from build123d import *
from build123d import SkipClean  # not in build123d's __all__

# Parameters (mm, degrees)
F0_W             = 44.45
F0_H             = 25.4
F1_DEPTH         = 44.45
F2_W             = 12.7
F2_H             = 44.45
F3_DEPTH         = 12.7
F4_W             = 44.45
F4_H             = 12.7
F5_DEPTH         = 6.985
F7_D             = 12.7
F8_W             = 12.7
F8_H             = 6.35
F9_DEPTH         = 12.7
F9_COPIES2_COUNT = 2
F9_COPIES2_PITCH = 49.595085
F11_D            = 4.4958
F13_D            = 3.4544


# Not quite as in the source:
# - after a boolean that leaves OpenCascade's solid faulty, fix() repairs it
# - a length typed as a fraction of an inch, garbled in the dataset ("3 / 203.2 mm" for 3/8 in), is restored
# - a pattern or mirror of a feature is missing from the dataset's text; its kind, count and spacing are read off the source's solid


with BuildPart() as f1:
    # F0 (on Top) → F1 (new body)
    with BuildSketch(Plane.XY):
        Rectangle(F0_W, F0_H)
    extrude(amount=F1_DEPTH)

    # F2 (on face) → F3 (cut)
    with BuildSketch(Plane.XZ.offset(12.7)):
        with Locations((0, 22.225)):
            Rectangle(F2_W, F2_H)
    extrude(amount=-F3_DEPTH, mode=Mode.SUBTRACT)

    # F4 (on face) → F5 (cut)
    with BuildSketch(Plane(origin=(0, 12.7, 0), x_dir=(-1, 0, 0), z_dir=(0, 1, 0))):
        with Locations((0, 22.225)):
            Rectangle(F4_W, F4_H)
    extrude(amount=-F5_DEPTH, mode=Mode.SUBTRACT)

    # F7 (through all)
    with Locations(Plane.XZ.offset(12.7)):
        with Locations((0, 22.225)):
            Hole(F7_D / 2)

    # F8 (on face) → F9 (join)
    with BuildSketch(Plane(origin=(0, 12.7, 0), x_dir=(-1, 0, 0), z_dir=(0, 1, 0))):
        with Locations((15.875, 3.175)):
            Rectangle(F8_W, F8_H)
    f9 = extrude(amount=F9_DEPTH)

    # F9_copies: F9 across plane
    add(f9.mirror(Plane(origin=(0, 0, 0), x_dir=(0, 0, -1), z_dir=(0, -1, 0))), clean=False)

    # F9_copies1: F9 across plane
    add(f9.mirror(Plane(origin=(0, 0, 0), x_dir=(0, 0, 1), z_dir=(1, 0, 0))), clean=False)

    # F9_copies2: F9 ×2
    with SkipClean():  # cleaning this boolean's faces spoils the solid; the shape is the same uncleaned
        with Locations(*[Vector(0.6401843997, -0.7682212796, 0) * (i * F9_COPIES2_PITCH) for i in range(1, F9_COPIES2_COUNT)]):
            add(f9, clean=False)

    # F11 (through all)
    with Locations(Plane.XY.offset(6.35)):
        with Locations((-15.875, 19.05)):
            f11 = Hole(F11_D / 2)

    add(f1.part.fix(), mode=Mode.REPLACE)

    # F11_copies: F11 across plane
    add(f11.mirror(Plane(origin=(0, 0, 0), x_dir=(0, 0, -1), z_dir=(0, -1, 0))), clean=False, mode=Mode.SUBTRACT)

    # F11_copies1: F11 across plane
    add(f11.mirror(Plane(origin=(0, 0, 0), x_dir=(0, 0, 1), z_dir=(1, 0, 0))), clean=False, mode=Mode.SUBTRACT)

    # F11_copies2: F11 across plane
    add(f11.mirror(Plane(origin=(0, 0, 0), x_dir=(-0.7682212796, -0.6401843997, 0), z_dir=(0.6401843997, -0.7682212796, 0))), clean=False, mode=Mode.SUBTRACT)

    # F13 (through all)
    with Locations(Plane.XZ.offset(12.7)):
        with Locations((-12.7, 31.75), (12.7, 12.7)):
            Hole(F13_D / 2)


solid = f1.part
Can you work these out from the model? Positions are in its coordinate system, mm. A direction names the side the tool comes from. Give positions to 0.01 mm unless a question says otherwise; leave off trailing zeros. Write each loop counter-clockwise with the first axis right and the second up, starting at its lowest first coordinate (ties: lowest second). Pieces come first, ordered by that corner, then holes. Notation, with made-up numbers: (60, 36.5) -> (78, 36.5) arc R6 ccw to (78, 42.5) -> close; hole circle Ø8 at (85.25, -36.75). An arc over 180 degrees is marked (long way). Answer as a JSON object with one key per item and string values. Group by question number.
Item 1: I'm going to push flat-ended pins straight in: P1, Ø12, axis at x = -14.5, z = 35, coming from the -Y side; P2, Ø14, axis at x = 18.5, y = 21, coming from the +Z side; P3, Ø5.5, axis at x = 12.7, z = 12.7, coming from the +Y side. Where does each tip first touch, or does it pass through?
Item 2: Suppose I cut it at C-C (y = -14.5). Please give me the cut outline in (x, z) (3 decimals).
Item 3: Suppose I cut it at D-D (z = 36.5). Please give me the cut outline in (x, y) (3 decimals).
Item 4: Please list where these lines run through material, in increasing order: line 1 (X direction, y = -19, z = 4) (3 decimals); line 2 (X direction, y = -7, z = 35.5) (3 decimals); line 3 (Z direction, x = -3.5, y = 10) (3 decimals). Write a range as [from, to].
Item 5: We'd pull the mould along Y, two halves only. Please class faces 5 (the face through (17.95, 18.19, 3.13)), 6 (the face through (-16, -25.4, 3)), 7 (the face through (0, 9, 15.875)): +Y half, -Y half, draft (parallel to the pull), parting line (faces both ways), or undercut.
Item 6: Suppose I cut it at A-A (z = 12.7). Please give me the cut outline in (x, y) (3 decimals), plus the area to 3 significant figures.
Item 7: Suppose I cut it at B-B (x = -12.7). Please give me the cut outline in (y, z) (3 decimals), plus the area to 3 significant figures.
Item 8: For faces 1 (the face through (-17.95, 18.19, 3.13)), 2 (the face through (9.525, -19, 3)), 3 (the face through (13, -19, 6.35)), 4 (the face through (-13, 5.715, 22)), which set-ups out of +Z, -Z, +X, -X, +Y, -Y let a thin tool reach every point of the face, with its end or its side?
Findings:
{
 "1": {"P1": "stops at y = -12.7", "P2": "stops at z = 6.35", "P3": "stops at y = 12.7"},
 "2": {"outline": "(-22.225, 0) -> (-9.525, 0) -> (-9.525, 6.35) -> (-22.225, 6.35) -> close; (9.525, 0) -> (22.225, 0) -> (22.225, 6.35) -> (9.525, 6.35) -> close"},
 "3": {"outline": "(-22.225, -12.7) -> (-6.35, -12.7) -> (-6.35, 0) -> (6.35, 0) -> (6.35, -12.7) -> (22.225, -12.7) -> (22.225, 12.7) -> (-22.225, 12.7) -> close"},
 "4": {"line 1": "x = [-22.225, -18.122], [-13.628, -9.525], [9.525, 13.628], [18.122, 22.225]", "line 2": "x = [-22.225, -6.35], [6.35, 22.225]", "line 3": "z = [0, 15.875], [28.575, 44.45]"},
 "5": {"face 5": "undercut", "face 6": "-Y half", "face 7": "draft"},
 "6": {"outline": "(-22.225, -12.7) -> (-6.35, -12.7) -> (-6.35, 0) -> (6.35, 0) -> (6.35, -12.7) -> (10.973, -12.7) -> (10.973, 12.7) -> (-22.225, 12.7) -> close; (14.427, -12.7) -> (22.225, -12.7) -> (22.225, 12.7) -> (14.427, 12.7) -> close", "area": "880 mm²"},
 "7": {"outline": "(-25.4, 0) -> (25.4, 0) -> (25.4, 6.35) -> (12.7, 6.35) -> (12.7, 15.875) -> (5.715, 15.875) -> (5.715, 28.575) -> (12.7, 28.575) -> (12.7, 30.023) -> (-12.7, 30.023) -> (-12.7, 6.35) -> (-25.4, 6.35) -> close; (-12.7, 33.477) -> (12.7, 33.477) -> (12.7, 44.45) -> (-12.7, 44.45) -> close", "area": "1,110 mm²"},
 "8": {"face 1": "+Z, -Z", "face 2": "+Z, -Z, -Y", "face 3": "+Z, +X, -X, -Y", "face 4": "+X, -X, +Y"}
}
